from build123d import *

# Parameters (mm, degrees)
SKETCH2_R               = 2.5
CUT_EXTRUDE1_DEPTH      = 6
CUT_EXTRUDE1_DEPTH_BACK = 6
SKETCH4_W               = 12
SKETCH4_H               = 18
CUT_EXTRUDE2_DEPTH      = 1.830127
SKETCH3_R               = 3
SKETCH3_R_2             = 2.5
EXTRUDE_THIN1_DEPTH     = 3.75


with BuildPart() as part:
    # Sketch1 → Revolve1 (revolve)
    with BuildSketch(Plane.XY):
        with BuildLine():
            Line((0, 0), (0, -7))
            Line((0, -7), (1.75, -7))
            Line((1.75, -7), (1.75, -17))
            Line((1.75, -17), (3.5, -17))
            Line((3.5, -17), (3.5, -3.570714214))
            ThreePointArc((3.5, -3.570714214), (4.628907596, 1.890294809), (0, 5))
            Line((0, 5), (0, 0))
        make_face()
    revolve(axis=Axis((0, 0, 0), (0, 1, 0)))

    # Sketch2 → Cut-Extrude1 (cut, two sides)
    with BuildSketch(Plane.XY) as cut_extrude1_sk:
        Circle(SKETCH2_R)
    extrude(amount=CUT_EXTRUDE1_DEPTH, mode=Mode.SUBTRACT)
    extrude(cut_extrude1_sk.sketch, amount=-CUT_EXTRUDE1_DEPTH_BACK, mode=Mode.SUBTRACT)

    # Sketch4 → Cut-Extrude2 (cut)
    with BuildSketch(Plane.XY.offset(2.5)):
        Rectangle(SKETCH4_W, SKETCH4_H)
    cut_extrude2 = extrude(amount=CUT_EXTRUDE2_DEPTH, mode=Mode.SUBTRACT)

    # Mirror1: Cut-Extrude2 across plane
    add(cut_extrude2.mirror(Plane.XY), mode=Mode.SUBTRACT)

    # Sketch3 → Extrude-Thin1 (add, symmetric)
    with BuildSketch(Plane.XY):
        Circle(SKETCH3_R)
        Circle(SKETCH3_R_2, mode=Mode.SUBTRACT)
    extrude(amount=EXTRUDE_THIN1_DEPTH, both=True)


solid = part.part
Verification items for the finished model (mm, model axes). A direction names the side the tool comes from. Give positions to 0.01 mm unless a question says otherwise; leave off trailing zeros. Loops run counter-clockwise (first coordinate to the right, second up) from the corner with the lowest first, then second, coordinate; pieces in that order, holes last.
1) Sectioned sample at B-B, the plane x = 0. Enter the section's corners in (y, z).
2) Set-up check for faces 4 (the cylindrical face through (-3, 0, -3)), 5 (the flat face through (0, -9, -3)), 6 (the flat face through (-2, 2, 3.75)), 7 (the cylindrical face through (-3, 0, 3)), 8 (the cylindrical face through (1.617, -12.07, 0.67)): record each of +Z, -Z, +X, -X, +Y, -Y from which the full face is reachable in a straight line by a thin tool's end or side.
3) Sectioned sample at D-D, the plane z = 0. Enter the section's corners in (x, y).
4) Draft check along Y on faces 1 (the flat face through (0, -7, 0)), 2 (the flat face through (-2, 2, -3.75)), 3 (the flat face through (0, -9, 3)). Enter one of: pulls with the +Y half, pulls with the -Y half, needs draft (parallel to the pull), parting line crosses it, or undercut.
5) Thickness scan on line 1 along X through (y, z) = (-13.25, 0); line 2 along Y through (x, z) = (-0.25, 3). Record the ranges inside material, lowest first.
6) Sectioned sample at A-A, the plane y = 0. Enter the section's corners in (x, z).
7) Depth check by flat-ended pin: pin 1 Ø1 at (x, y) = (-1.5, -14) entering from +Z; pin 2 Ø1.5 at (y, z) = (2, 0.5) entering from -X; pin 3 Ø0.8 at (x, z) = (0, 3) entering from +Y. Enter the tip coordinate at first touch or a pass-through.
8) Sectioned sample at C-C, the plane z = -2.75. Enter the section's corners in (x, y).
Answers:
1. outline: (-17, -3.5) - (-9, -3.5) - (-9, -2.5) - (-3, -2.5) - (-3, -3.75) - (-2.5, -3.75) - (-2.5, 3.75) - (-3, 3.75) - (-3, 2.5) - (-9, 2.5) - (-9, 3.5) - (-17, 3.5) - (-17, 1.75) - (-7, 1.75) - (-7, -1.75) - (-17, -1.75) - close; (2.5, -3.75) - (3, -3.75) - (3, -2.5) - (4.33, -2.5) arc R5 ccw to (4.33, 2.5) - (3, 2.5) - (3, 3.75) - (2.5, 3.75) - close
2. face 4: -Z
2. face 5: -Z, +X, -X
2. face 6: +Z, +X, -X, +Y, -Y
2. face 7: +Z
2. face 8: -Y
3. outline: (-3.5, -17) - (-1.75, -17) - (-1.75, -7) - (1.75, -7) - (1.75, -17) - (3.5, -17) - (3.5, -3.57) arc R5 ccw (long way) to (-3.5, -3.57) - close; hole circle Ø5 at (0, 0)
4. face 1: pulls with the -Y half
4. face 2: needs draft
4. face 3: undercut
5. line 1: x = -3.5 to -1.75, 1.75 to 3.5
5. line 2: y = -17 to -9, -2.99 to -2.49, 2.49 to 2.99
6. outline: (-4.33, -2.5) - (-3, -2.5) - (-3, -3.75) - (-2.5, -3.75) - (-2.5, 3.75) - (-3, 3.75) - (-3, 2.5) - (-4.33, 2.5) arc R5 ccw to start; (2.5, -3.75) - (3, -3.75) - (3, -2.5) - (4.33, -2.5) arc R5 ccw to (4.33, 2.5) - (3, 2.5) - (3, 3.75) - (2.5, 3.75) - close
7. pin 1: stops at z = 3.35
7. pin 2: stops at x = -4.82
7. pin 3: stops at y = 3
8. outline: circle Ø6 at (0, 0); (-2.17, -17) - (2.17, -17) - (2.17, -9) - (-2.17, -9) - close; hole circle Ø5 at (0, 0)
